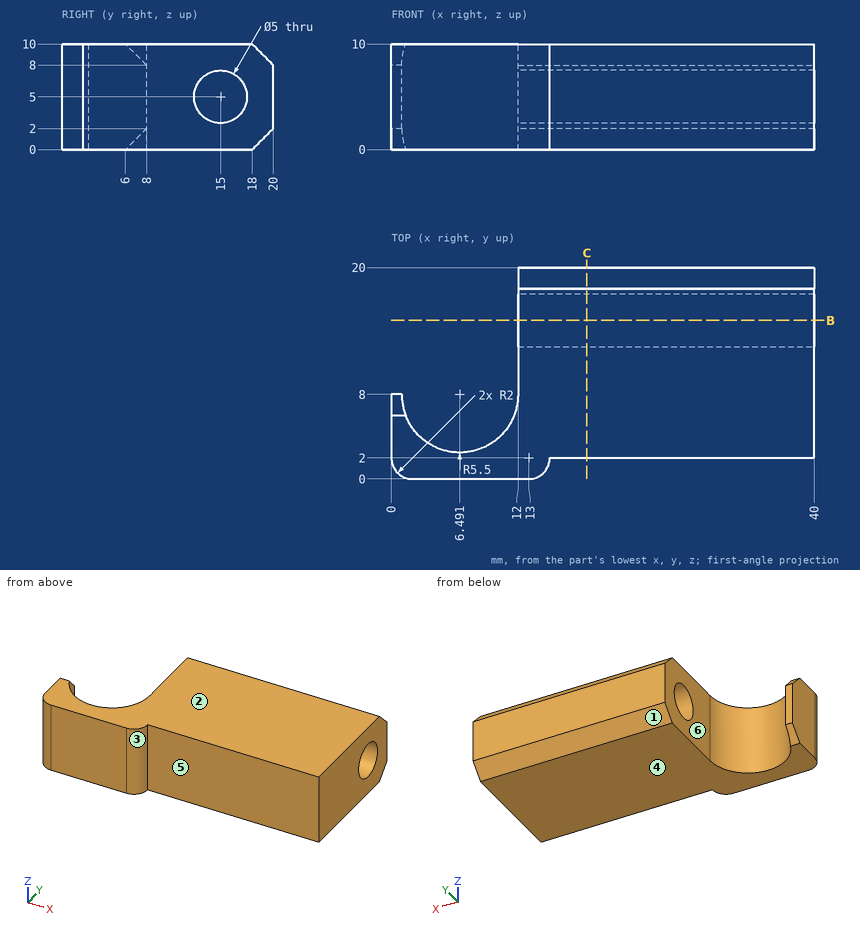
Design review of the part shown in the three views and the two pictorial views. Dimensions are in mm from the part's minimum x, y and z. A direction names the side the tool comes from. Give positions to 0.01 mm unless a question says otherwise; leave off trailing zeros. Loops run counter-clockwise (first coordinate to the right, second up) from the corner with the lowest first, then second, coordinate; pieces in that order, holes last. Notation, with made-up numbers: M -40,-17.75 L -8,-17.75 A24 ccw -8,19.25 Z; hole C 26,78.25 d2. An arc over 180 degrees is marked long. Answer as a JSON object with one key per item and string values. Group by question number.
Q1. Tool access review of the marked faces 4, 5 and 6: name each direction out of +Z, -Z, +X, -X, +Y, -Y from which nothing blocks a thin tool from reaching the whole face with its end or side.
Q2. Mouldability with a two-part tool opening along Y and no side actions: class the marked faces 1, 2 and 3 as +Y half, -Y half, draft (parallel to the pull), parting line (faces both ways), or undercut.
Q3. For probe 1 along Z at (x, y) = (18, 15); probe 2 along X at (y, z) = (5.75, 6.5); probe 3 along X at (y, z) = (5, 3), list the stretches that pass through material, from the lowest coordinate up. Write a range as [from, to].
Q4. Add section C-C on x = 18.5. Give the boundary of the cut face in (y, z).
Q5. Insertion check: P1, Ø3, axis at x = 27, z = 3.5, coming from the -Y side; P2, Ø3, axis at x = 11.5, y = 9.5, coming from the -Z side; P3, Ø8, axis at x = 5, y = 10.5, coming from the +Z side; P4, Ø0.8, axis at x = 0.5, z = 6, coming from the +Y side. Each pin has a flat end and moves straight along its axis. Give the tip position at first contact, or say it passes through.
Q6. Add section B-B on y = 15. Give the boundary of the cut face in (x, z), and give its area (3 significant figures).
Checked values:
{
 "1": {"face 4": "-Z, +X, -X, +Y, -Y", "face 5": "+Z, -Z, +X, -Y", "face 6": "+Z, -Z, -X, +Y"},
 "2": {"face 1": "+Y half", "face 2": "draft", "face 3": "-Y half"},
 "3": {"probe 1": "[0, 2.5], [7.5, 10]", "probe 2": "[0, 1.47], [11.51, 40]", "probe 3": "[0, 1.88], [11.1, 40]"},
 "4": {"outline": "M 2,0 L 18,0 L 20,2 L 20,8 L 18,10 L 2,10 Z; hole C 15,5 d5"},
 "5": {"P1": "y = 2", "P2": "z = 0", "P3": "through", "P4": "y = 8"},
 "6": {"outline": "M 12,0 L 40,0 L 40,2.5 L 12,2.5 Z; M 12,7.5 L 40,7.5 L 40,10 L 12,10 Z", "area": "140 mm²"}
}
